Could you check a few things on this drawing? It's one solid part, dimensions in mm from its lowest x, y, z. A direction names the side the tool comes from. Give positions to 0.01 mm unless a question says otherwise; leave off trailing zeros. Loops run counter-clockwise (first coordinate to the right, second up) from the corner with the lowest first, then second, coordinate; pieces in that order, holes last.
1. For P1, Ø1, axis at y = 26.5, z = 52.5, coming from the -X side; P2, Ø1.8, axis at x = 2, z = 49.5, coming from the -Y side; P3, Ø2, axis at x = 5.5, z = 33, coming from the -Y side (1 decimal); P4, Ø1, axis at x = 5, z = 35.5, coming from the -Y side (1 decimal), each with a flat end and sliding along its axis, tell me the tip position at first contact or that it passes through.
2. For the marked faces 1 and 2, which set-ups out of +Z, -Z, +X, -X, +Y, -Y let a thin tool reach every point of the face, with its end or its side?
3. Imagine slicing it at D-D (y = 4.5). List the corners of the cut face in (x, z) for me (1 decimal), plus the area to 3 significant figures.
4. Imagine slicing it at C-C (z = 53). List the corners of the cut face in (x, y) for me.
5. I need wall thicknesses on line 1 along Y through (x, z) = (2.75, 47.5); line 2 along X through (y, z) = (24.5, 41); line 3 along Y through (x, z) = (5, 20). Which ranges of each line are inside material? Lowest first, please.
6. Thinking about a two-plate mould opening in Z: for the marked faces 3, 4 and 5, which applies, +Z half, -Z half, draft (parallel to the pull), parting line (faces both ways), or undercut?
7. Imagine slicing it at A-A (y = 24). List the corners of the cut face in (x, z) for me (1 decimal).
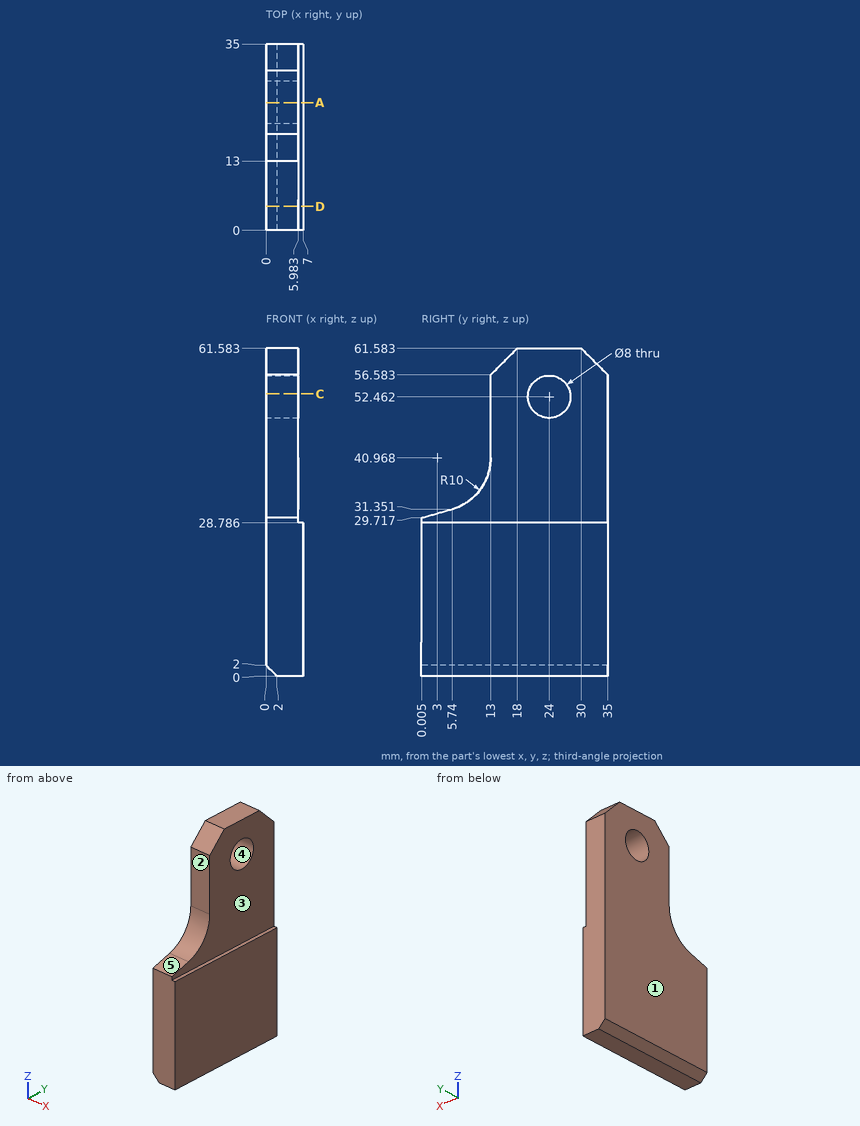
Derived:
1. P1: passes through
1. P2: stops at y = 13
1. P3: stops at y = 7.4
1. P4: stops at y = 11
2. face 1: +Z, -Z, -X, +Y, -Y
2. face 2: +Z, +X, -X, -Y
3. outline: (0, 2) - (2, 0) - (7, 0) - (7, 28.8) - (6, 28.8) - (6, 31) - (0, 31) - close
3. area: 213 mm2
4. outline: (0, 13) - (5.98, 13) - (5.98, 20.04) - (0, 20.04) - close; (0, 27.96) - (5.98, 27.96) - (5.98, 35) - (0, 35) - close
5. line 1: y = 13 to 35
5. line 2: x = 0 to 5.98
5. line 3: y = 0 to 35
6. face 3: draft
6. face 4: undercut
6. face 5: +Z half
7. outline: (0, 2) - (2, 0) - (7, 0) - (7, 28.8) - (6, 28.8) - (6, 48.5) - (0, 48.5) - close; (0, 56.5) - (6, 56.5) - (6, 61.6) - (0, 61.6) - close
